For this review, use the dimensioned drawing (mm, ordinates from the lowest corner) and the shaded views. A direction names the side the tool comes from. Give positions to 0.01 mm unless a question says otherwise; leave off trailing zeros. Write each loop counter-clockwise with the first axis right and the second up, starting at its lowest first coordinate (ties: lowest second). Pieces come first, ordered by that corner, then holes. Notation, with made-up numbers: M -2,0.25 L 21,0.25 A15 ccw 21,11.25 Z; hole C 6.25,-4.5 d9. An arc over 180 degrees is marked long. Write each question's results on one line, items separated by ' | '. Start each with the question number.
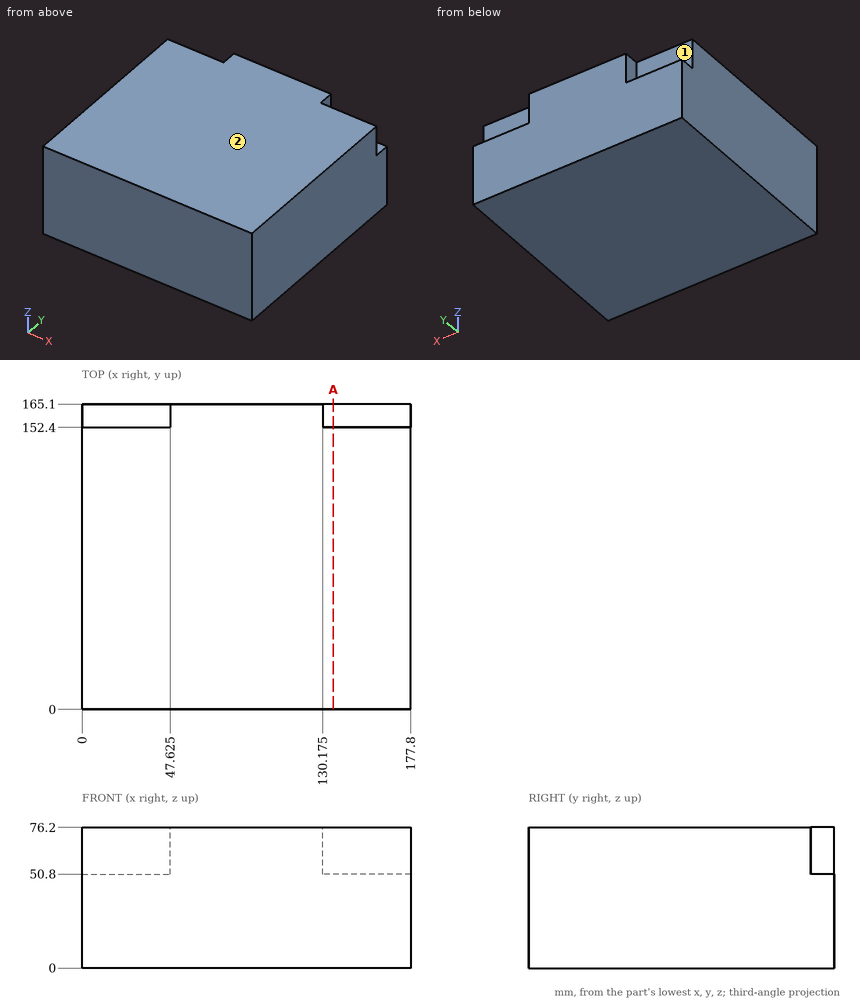
(1) Wall thickness on L1, parallel to Y at x = 134.5, z = 62: over which ranges is the line inside the solid? List them lowest first.
(2) Clearance check with flat-ended pins moving along their axes: P1, Ø10, axis at x = 17.5, y = 157.5, coming from the +Z side; P2, Ø6.5, axis at y = 159.5, z = 63.5, coming from the -X side (3 decimals); P3, Ø12.5, axis at x = 155, z = 61.5, coming from the +Y side. State where each tip first meets the part, or that it passes through.
(3) Add section A-A (x = 136). State the section outline as (y, z) points.
(4) Machinability: for the marked faces 1 and 2, which of the approach directions +Z, -Z, +X, -X, +Y, -Y give a long, thin tool a straight path to every point of the face, cutting with its end or side? Answer none if there is none.
Calculated:
1) L1: y = 0 to 152.4
2) P1: stops at z = 50.8 | P2: stops at x = 47.625 | P3: stops at y = 152.4
3) outline: M 0,0 L 165.1,0 L 165.1,50.8 L 152.4,50.8 L 152.4,76.2 L 0,76.2 Z
4) face 1: +Z, -X, +Y | face 2: +Z, +X, -X, +Y, -Y
